Check sheet for the modelled part. Datum: model origin and axes. Units: mm. A direction names the side the tool comes from. Round coordinates to 2 decimals unless told otherwise and drop trailing zeros. Loops run counter-clockwise (first coordinate to the right, second up) from the corner with the lowest first, then second, coordinate; pieces in that order, holes last. Notation, with made-up numbers: (9.25, -9.75) - (43.25, -9.75) arc R29 ccw to (43.25, 17.25) - close; hole circle Ø8 at (-30, -0.5). An arc over 180 degrees is marked (long way). Return JSON: item names as keys, results as strings.
from build123d import *

# Parameters (mm, degrees)
EXTRUDE_1_DEPTH     = 45
SKETCH_2_R          = 1.5
CUT_EXTRUDE_1_DEPTH = 50.309633947
SKETCH_3_R          = 1.5
CUT_EXTRUDE_2_DEPTH = 50.915785078


with BuildPart() as part:
    # 草图1 → 凸台-拉伸1 (new body)
    with BuildSketch(Plane.XY):
        Polygon((-8.16, 16.2), (-6.16, 16.2), (-6.16, -1.8), (3.84, -1.8), (3.84, -3.8), (-8.16, -3.8), align=None)
    extrude(amount=EXTRUDE_1_DEPTH)

    # 草图2 → 切除-拉伸1 (cut, through all)
    with BuildSketch(Plane.ZY.offset(8.16)):
        with Locations((4, 6.2)):
            Circle(SKETCH_2_R)
        with Locations(Location((41, 6.2, 0), (0, 0, 270))):
            Circle(SKETCH_2_R)
    extrude(amount=-CUT_EXTRUDE_1_DEPTH, mode=Mode.SUBTRACT)

    # 草图3 → 切除-拉伸2 (cut, through all)
    with BuildSketch(Plane.XZ.offset(3.8)):
        with Locations((-1.16, 33)):
            Circle(SKETCH_3_R)
        with Locations((-1.16, 12)):
            Circle(SKETCH_3_R)
    extrude(amount=-CUT_EXTRUDE_2_DEPTH, mode=Mode.SUBTRACT)


solid = part.part
Q1. Sectioned sample at D-D (y = -2.5). Enter the section's corners in (x, z).
Answer key:
{"outline": "(-8.16, 0) - (3.84, 0) - (3.84, 45) - (-8.16, 45) - close; hole circle Ø3 at (-1.16, 12); hole circle Ø3 at (-1.16, 33)"}
Q2. Draft check along X on faces 3 (the face through (-7, 3, 45)), 4 (the face through (-6.16, 7, 22)), 5 (the face through (-1.485, -2.814, 31.536)), 6 (the face through (0.226, -2.814, 11.425)). Enter one of: released by +X, released by -X, zero draft, split by the parting line, or undercut.
Answer key:
{"face 3": "zero draft", "face 4": "released by +X", "face 5": "undercut", "face 6": "undercut"}
Q3. Tool access check on faces 1 (the face through (-7.17, 4.87, 4.69)), 2 (the face through (-1, -1.8, 22)). Record the directions out of +Z, -Z, +X, -X, +Y, -Y that give a thin tool (end or side, any length) a straight path to the whole face; none if there is none.
Answer key:
{"face 1": "+X, -X", "face 2": "+Z, -Z, +X, +Y"}
Q4. Scan lines: probe 1 along Z at (x, y) = (-1.16, -2.55); probe 2 along Y at (x, z) = (-6.75, 4); probe 3 along X at (y, z) = (2, 40). Record each from-to range of solid material in increasing order. Write a range as [from, to].
Answer key:
{"probe 1": "z = [0, 10.5], [13.5, 31.5], [34.5, 45]", "probe 2": "y = [-3.8, 4.7], [7.7, 16.2]", "probe 3": "x = [-8.16, -6.16]"}
Q5. Sectioned sample at B-B (z = 13). Enter the section's corners in (x, y), plus the area to 3 significant figures.
Answer key:
{"outline": "(-8.16, -3.8) - (-2.28, -3.8) - (-2.28, -1.8) - (-6.16, -1.8) - (-6.16, 16.2) - (-8.16, 16.2) - close; (-0.04, -3.8) - (3.84, -3.8) - (3.84, -1.8) - (-0.04, -1.8) - close", "area": "55.5 mm²"}
Q6. Sectioned sample at A-A (y = 6.2). Enter the section's corners in (x, z).
Answer key:
{"outline": "(-8.16, 0) - (-6.16, 0) - (-6.16, 2.5) - (-8.16, 2.5) - close; (-8.16, 5.5) - (-6.16, 5.5) - (-6.16, 39.5) - (-8.16, 39.5) - close; (-8.16, 42.5) - (-6.16, 42.5) - (-6.16, 45) - (-8.16, 45) - close"}
Q7. Sectioned sample at C-C (x = -7.5). Enter the section's corners in (y, z), plus the area to 3 significant figures.
Answer key:
{"outline": "(-3.8, 0) - (16.2, 0) - (16.2, 45) - (-3.8, 45) - close; hole circle Ø3 at (6.2, 4); hole circle Ø3 at (6.2, 41)", "area": "886 mm²"}
Q8. Depth check by flat-ended pin: P1, Ø3.5, axis at x = -1.16, z = 33, coming from the +Y side; P2, Ø10, axis at y = 4.5, z = 36, coming from the +X side. Enter the tip coordinate at first touch or a pass-through.
Answer key:
{"P1": "stops at y = -1.8", "P2": "stops at x = -6.16"}
